```python
from build123d import *

# Parameters (mm, degrees)
SALIENTE_EXTRUIR1_DEPTH = 1.25
SALIENTE_EXTRUIR2_DEPTH = 3.25
SALIENTE_EXTRUIR3_DEPTH = 219.699982554
SALIENTE_EXTRUIR4_DEPTH = 5
REDONDEO1_R             = 0.5
CROQUIS7_R              = 1.65
CORTAR_EXTRUIR1_DEPTH   = 409.725190141


with BuildPart() as part:
    # Croquis1 → Saliente-Extruir1 (new body)
    with BuildSketch(Plane.XY):
        Polygon((76.151803136, 59.751000255), (76.151803136, 266.850888729), (276.149988174, 266.850888729), (276.149988174, 59.751000255), (287.750005722, 59.751000255), (287.750005722, 290.251016617), (92.349797487, 290.251016617), (92.349797487, 279.450982809), (64.949996769, 279.450982809), (64.439042354, 59.751000255), align=None)
    extrude(amount=SALIENTE_EXTRUIR1_DEPTH)

    # Croquis3 → Saliente-Extruir2 (add)
    with BuildSketch(Plane.XY.offset(1.25)):
        Polygon((65.549881, 59.751000255), (65.549881, 277.83340256), (286.749988794, 277.845112205), (286.751151675, 59.751000255), (287.750005722, 59.751000255), (287.750005722, 279.450982809), (92.349797487, 279.450982809), (64.949996769, 279.450982809), (64.439042354, 59.751000255), align=None)
    extrude(amount=SALIENTE_EXTRUIR2_DEPTH)

    # Croquis4 → Saliente-Extruir3 (add)
    with BuildSketch(Plane(origin=(0, 279.450982809, 0), x_dir=(1, 0, 0), z_dir=(0, 1, 0))):
        with BuildLine():
            Line((64.20314146, -3.994108901), (64.439042354, -4.5))
            Line((64.439042354, -4.5), (64.949996769, -4.5))
            Line((64.949996769, -4.5), (64.949996769, 0))
            Line((64.949996769, 0), (64.159257759, 0))
            ThreePointArc((64.159257759, 0), (62.250455442, -2.018267743), (64.20314146, -3.994108901))
        make_face()
    extrude(amount=-SALIENTE_EXTRUIR3_DEPTH)

    # Croquis6 → Saliente-Extruir4 (add)
    with BuildSketch(Plane(origin=(0, 279.450982809, 0), x_dir=(1, 0, 0), z_dir=(0, 1, 0))):
        with BuildLine():
            Line((67.471777384, 0), (64.029912079, 0))
            ThreePointArc((64.029912079, 0), (65.750844731, -3.019014625), (67.471777384, 0))
        make_face()
    extrude(amount=SALIENTE_EXTRUIR4_DEPTH)

    # Redondeo1
    redondeo1_edges = [part.edges().sort_by_distance(p)[0] for p in [
        (65.757057169, 279.450982809, 3.019004976),
    ]]
    fillet(redondeo1_edges, radius=REDONDEO1_R)

    # Croquis7 → Cortar-Extruir1 (cut, through all)
    with BuildSketch(Plane.XY.offset(1.25)):
        with Locations((70.850842068, 74.751000255)):
            Circle(CROQUIS7_R)
        with Locations((70.850842068, 251.850888729)):
            Circle(CROQUIS7_R)
        with Locations((70.850842068, 221.850888729)):
            Circle(CROQUIS7_R)
        with Locations((70.850842068, 148.300944492)):
            Circle(CROQUIS7_R)
        with Locations((91.151803136, 272.342426261)):
            Circle(CROQUIS7_R)
        with Locations((176.149949567, 272.342426261)):
            Circle(CROQUIS7_R)
        with Locations((261.148095998, 272.342426261)):
            Circle(CROQUIS7_R)
        with Locations((281.449057067, 251.850888729)):
            Circle(CROQUIS7_R)
        with Locations((281.449057067, 221.850888729)):
            Circle(CROQUIS7_R)
        with Locations((281.449057067, 148.300944492)):
            Circle(CROQUIS7_R)
        with Locations((281.449057067, 74.751000255)):
            Circle(CROQUIS7_R)
    extrude(amount=-CORTAR_EXTRUIR1_DEPTH, mode=Mode.SUBTRACT)


solid = part.part
```
The listing builds one solid part. Answer for the finished solid, in the listing's coordinates (mm). Give positions to 0.01 mm unless a question says otherwise; leave off trailing zeros. Write each loop counter-clockwise with the first axis right and the second up, starting at its lowest first coordinate (ties: lowest second). Pieces come first, ordered by that corner, then holes. Notation, with made-up numbers: M 24.5,26.5 L 61.5,26.5 A21 ccw 61.5,61.5 Z; hole C -10.5,73.25 d6. An arc over 180 degrees is marked long. Write each question's results on one line, items separated by ' | '.
Q1. For a pull along X with two mould halves and no side action, classify faces 1 (the flat face through (168, 268, 0)), 2 (the flat face through (175.6, 274.3, 1.25)) as released by +X, released by -X, zero draft, split by the parting line, or undercut.
Output values:
face 1: zero draft | face 2: undercut
Q2. Section B-B, the plane x = 207.5 is taken. Write down the section's boundary in (y, z).
Output values:
outline: M 266.85,0 L 290.25,0 L 290.25,1.25 L 279.45,1.25 L 279.45,4.5 L 277.84,4.5 L 277.84,1.25 L 266.85,1.25 Z
Q3. Flat-ended cylindrical pins translate along their axes: P1, Ø1.4, axis at x = 192.5, z = 0.5, coming from the -Y side; P2, Ø1.5, axis at x = 65, z = 1.5, coming from the +Y side; P3, Ø2.5, axis at x = 91.15, y = 272.34, coming from the +Z side; P4, Ø1, axis at x = 134.5, z = 2.5, coming from the +Y side. Find the tip coordinate at first contact, or state that the pin passes through.
Output values:
P1: y = 266.85 | P2: y = 284.45 | P3: through | P4: y = 279.45
Q4. Section A-A, the plane y = 245 is taken. Write down the section's boundary in (x, z).
Output values:
outline: M 64.16,0 L 76.15,0 L 76.15,1.25 L 65.55,1.25 L 65.55,4.5 L 64.44,4.5 L 64.2,3.99 A2 ccw Z; M 276.15,0 L 287.75,0 L 287.75,4.5 L 286.75,4.5 L 286.75,1.25 L 276.15,1.25 Z
Q5. Consider L1, parallel to X at y = 86, z = 1.95; L2, parallel to Y at x = 253, z = 1.75; L3, parallel to Y at x = 109, z = 1.1. Determine where each line is inside the solid, lowest interval first. Write a range as from..to.
Output values:
L1: 62.25..65.55, 286.75..287.75 | L2: 277.84..279.45 | L3: 266.85..290.25
